Drawing for the job (mm, zero at the part's lowest x, y, z). Coordinates: 2 decimals unless noted, no trailing zeros. Write each loop counter-clockwise with the first axis right and the second up, starting at its lowest first coordinate (ties: lowest second). Pieces come first, ordered by that corner, then holes. Notation, with made-up numbers: (4.25, 49) -> (50.25, 49) arc R24 ccw to (50.25, 67) -> close; hole circle Ø5 at (23.5, 82). An arc over 180 degrees is marked (long way). Write each question's results on one line, items separated by ' | '. Start each with the question number.
Q1. Drill centre lines: line 1 (Y direction, x = 25.5, z = 73.5) (1 decimal); line 2 (Z direction, x = 25, y = 21); line 3 (X direction, y = 53, z = 112) (1 decimal). Where is each one in solid material? Low to high.
Q2. Two-plate mould, pull along X, no slides. Class the marked faces 1, 2 and 3: released by +X, released by -X, zero draft, split by the parting line, or undercut.
Q3. Saw through at A-A on y = 52. Give the cut face in (x, z), and give its area (3 significant figures).
Q4. Saw through at C-C on z = 85. Give the cut face in (x, y) (1 decimal), and give its area (3 significant figures).
Q5. Saw through at B-B on x = 49. Give the cut face in (y, z).
Q6. Drop flat-ended pins along their axis: pin 1 Ø1 at (x, y) = (47, 14.5) entering from +Z; pin 2 Ø13 at (x, y) = (24, 61) entering from +Z; pin 3 Ø6 at (x, z) = (12.5, 102) entering from +Y (1 decimal); pin 4 Ø12 at (x, y) = (37.5, 20.5) entering from -Z. Give the stop position or say it passes through.
Q7. Saw through at D-D on y = 38.5. Give the cut face in (x, z), and give its area (3 significant figures).
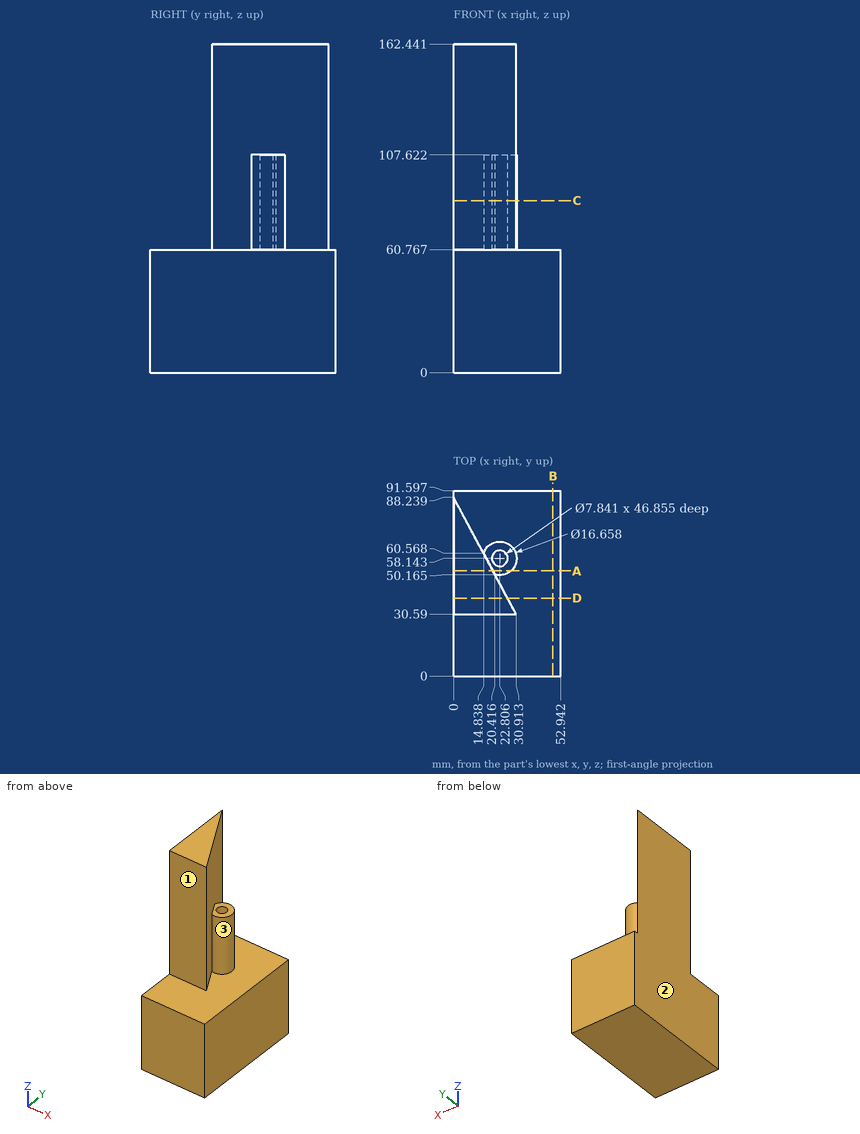
Returned:
1) line 1: y = 30.6 to 40.7, 50.3 to 55.3, 61 to 66 | line 2: z = 0 to 60.77 | line 3: x = 0 to 18.9
2) face 1: zero draft | face 2: released by -X | face 3: undercut
3) outline: (0, 0) -> (52.94, 0) -> (52.94, 60.77) -> (28.43, 60.77) -> (28.43, 107.62) -> (19.43, 107.62) -> (19.43, 162.44) -> (0, 162.44) -> close | area: 5,610 mm2
4) outline: (0, 30.6) -> (30.9, 30.6) -> (20.4, 50.2) arc R8.3 ccw (long way) to (14.8, 60.6) -> (0, 88.2) -> close; hole circle Ø7.8 at (22.8, 58.1) | area: 1,040 mm2
5) outline: (0, 0) -> (91.6, 0) -> (91.6, 60.77) -> (0, 60.77) -> close
6) pin 1: stops at z = 60.77 | pin 2: stops at z = 107.62 | pin 3: stops at y = 70.5 | pin 4: stops at z = 0
7) outline: (0, 0) -> (52.94, 0) -> (52.94, 60.77) -> (26.67, 60.77) -> (26.67, 162.44) -> (0, 162.44) -> close | area: 5,930 mm2
